from build123d import *

# Parameters (mm, degrees)
ESQUISSE1_R        = 1.6
BOSS_EXTRU_1_DEPTH = 3


with BuildPart() as part:
    # Esquisse1 → Boss.-Extru.1 (new body)
    with BuildSketch(Plane.XY.offset(3)):
        with BuildLine():
            Line((35, 3), (0, 3))
            ThreePointArc((0, 3), (-3, 0), (0, -3))
            Line((0, -3), (35, -3))
            ThreePointArc((35, -3), (38, 0), (35, 3))
        make_face()
        with Locations(Location((35, 0, 0), (0, 0, 180))):
            Circle(ESQUISSE1_R, mode=Mode.SUBTRACT)
        with Locations(Location((0, 0, 0), (0, 0, 180))):
            Circle(ESQUISSE1_R, mode=Mode.SUBTRACT)
    extrude(amount=-BOSS_EXTRU_1_DEPTH)


solid = part.part
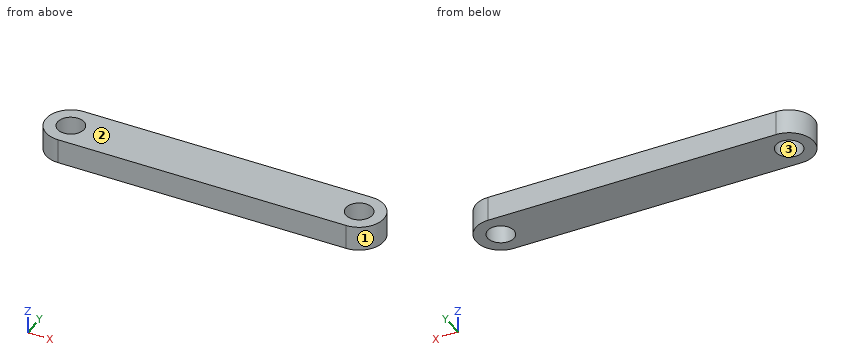
The model under review builds one solid part; all positions refer to its coordinate system, in mm. Face numbers are marked on the shaded views. Give positions to 0.01 mm unless a question says otherwise; leave off trailing zeros. Write each loop counter-clockwise with the first axis right and the second up, starting at its lowest first coordinate (ties: lowest second). Pieces come first, ordered by that corner, then holes. Notation, with made-up numbers: M 77,-25.75 L 101,-25.75 A23 ccw 101,-14.75 Z; hole C 27.25,28.5 d9. An arc over 180 degrees is marked long. One line per question, with ' | ' between items. Start each with the question number.
Item 1: We need section C-C on y = -2.3. Write out the cut boundary in (x, z).
Item 2: We need section B-B on z = 1.5. Write out the cut boundary in (x, y), plus the area to 3 significant figures.
Item 3: We need section A-A on y = 0. Write out the cut boundary in (x, z), plus the area to 3 significant figures.
Item 4: Wall thickness on line 1 (X direction, y = -0.1, z = 0.6); line 2 (Y direction, x = 35, z = 1.4); line 3 (X direction, y = 0.8, z = 2.1): over which ranges is each line inside the solid? List them lowest first. Write a range as from..to.
Item 5: Draft analysis for pull direction X (two halves, no side actions). For the marked faces 1, 2 and 3, state which applies: released by +X, released by -X, zero draft, split by the parting line, or undercut.
Results found:
1) outline: M -1.93,0 L 36.93,0 L 36.93,3 L -1.93,3 Z
2) outline: M 0,-3 L 35,-3 A3 ccw 35,3 L 0,3 A3 ccw Z; hole C 0,0 d3.2; hole C 35,0 d3.2 | area: 222 mm2
3) outline: M -3,0 L -1.6,0 L -1.6,3 L -3,3 Z; M 1.6,0 L 33.4,0 L 33.4,3 L 1.6,3 Z; M 36.6,0 L 38,0 L 38,3 L 36.6,3 Z | area: 104 mm2
4) line 1: x = -3..-1.6, 1.6..33.4, 36.6..38 | line 2: y = -3..-1.6, 1.6..3 | line 3: x = -2.89..-1.39, 1.39..33.61, 36.39..37.89
5) face 1: released by +X | face 2: zero draft | face 3: undercut
